Geometry: see drawing. Coordinates: mm, zero at the bounding-box minimum. Give positions to 0.01 mm unless a question says otherwise; leave off trailing zeros. Loops run counter-clockwise (first coordinate to the right, second up) from the corner with the lowest first, then second, coordinate; pieces in that order, holes last. Notation, with made-up numbers: (88, 87.5) - (131, 87.5) arc R29 ccw to (131, 114.5) - close; hole circle Ø2 at (-16.75, -39). An arc over 180 degrees is marked (long way). Use one line per item in the form item = value.
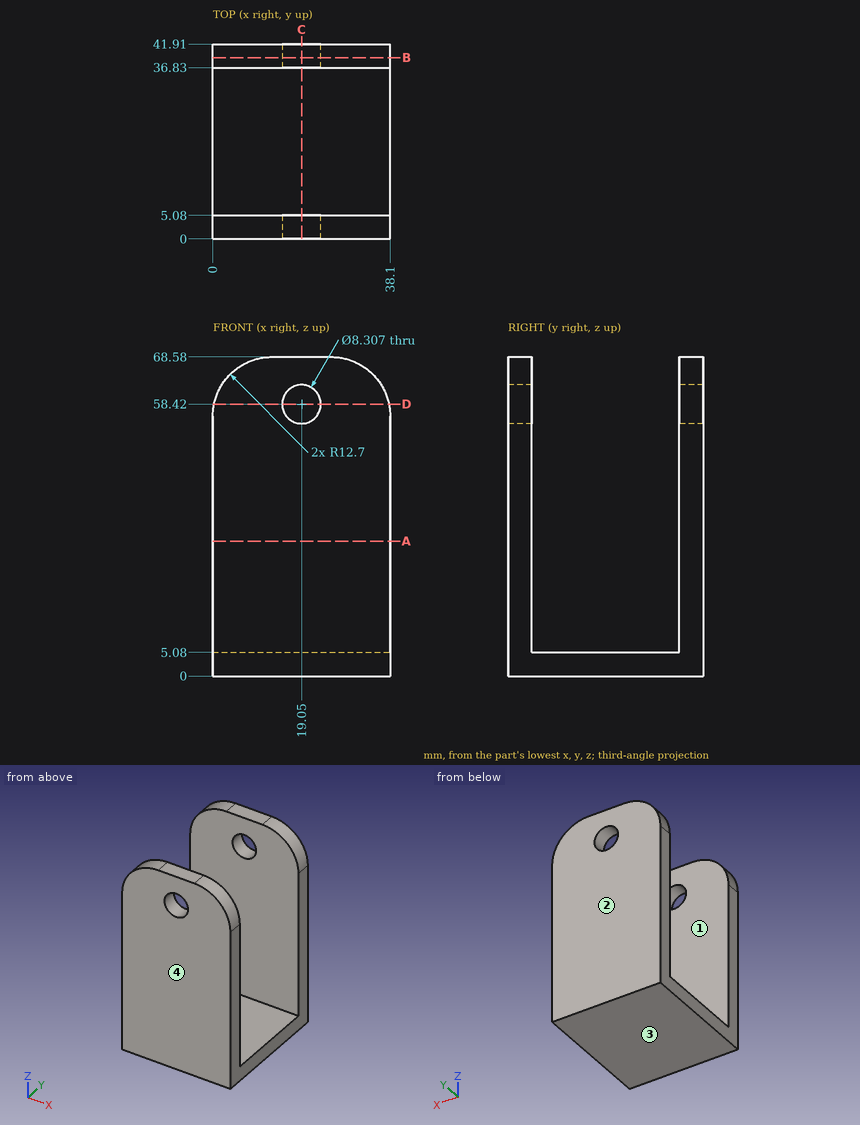
(1) Cut plane C-C (x = 19.05). Return the cut outline in (y, z).
Solution:
outline = (0, 0) - (41.91, 0) - (41.91, 54.27) - (36.83, 54.27) - (36.83, 5.08) - (5.08, 5.08) - (5.08, 54.27) - (0, 54.27) - close; (0, 62.57) - (5.08, 62.57) - (5.08, 68.58) - (0, 68.58) - close; (36.83, 62.57) - (41.91, 62.57) - (41.91, 68.58) - (36.83, 68.58) - close
(2) Cut plane B-B (y = 39). Return the cut outline in (x, z), plus the area to 3 significant figures.
Solution:
outline = (0, 0) - (38.1, 0) - (38.1, 55.88) arc R12.7 ccw to (25.4, 68.58) - (12.7, 68.58) arc R12.7 ccw to (0, 55.88) - close; hole circle Ø8.31 at (19.05, 58.42)
area = 2,490 mm2
(3) Material intervals for L1, parallel to Y at x = 2.5, z = 22.5; L2, parallel to Z at x = 19, y = 37; L3, parallel to Z at x = 12, y = 15.5, sorted ascending. Write a range as from..to.
Solution:
L1 = 0..5.08, 36.83..41.91
L2 = 0..54.27, 62.57..68.58
L3 = 0..5.08
(4) Cut plane D-D (z = 58.42). Return the cut outline in (x, y).
Solution:
outline = (0.26, 0) - (14.9, 0) - (14.9, 5.08) - (0.26, 5.08) - close; (0.26, 36.83) - (14.9, 36.83) - (14.9, 41.91) - (0.26, 41.91) - close; (23.2, 0) - (37.84, 0) - (37.84, 5.08) - (23.2, 5.08) - close; (23.2, 36.83) - (37.84, 36.83) - (37.84, 41.91) - (23.2, 41.91) - close
(5) Pin query (flat end, axial travel): P1, Ø16, axis at x = 17.5, y = 20.5, coming from the +Z side; P2, Ø8, axis at x = 7, y = 8, coming from the +Z side; P3, Ø11.5, axis at x = 16.5, z = 51.5, coming from the -Y side. Return the tip coordinate at first contact, or that it passes through.
Solution:
P1 = 5.08
P2 = 68.23
P3 = 0
(6) Pull-direction query (Y, two-part tool) for the marked faces 1, 2, 3 and 4; classes: released by +Y, released by -Y, zero draft, split by the parting line, or undercut.
Solution:
face_1 = undercut
face_2 = released by +Y
face_3 = zero draft
face_4 = released by -Y
(7) Cut plane A-A (z = 29). Return the cut outline in (x, y).
Solution:
outline = (0, 0) - (38.1, 0) - (38.1, 5.08) - (0, 5.08) - close; (0, 36.83) - (38.1, 36.83) - (38.1, 41.91) - (0, 41.91) - close
